Verification items for the finished model (mm, model axes). A direction names the side the tool comes from. Give positions to 0.01 mm unless a question says otherwise; leave off trailing zeros. Order: outer loops, then holes, each group sorted by start corner. A loop starts at its lowest first (then second) coordinate and runs counter-clockwise, first axis right, second up. Notation, with made-up numbers: (-22, 83.25) -> (7, 83.25) arc R24 ccw to (7, 97.25) -> close; hole circle Ø1 at (-18, -17). An arc over 180 degrees is marked (long way). Return JSON: item names as keys, results as strings. Group by question number.
(1) Cross-section at B-B on z = 88.5. Enter the section's corners in (x, y).
(2) Tool access check on faces 1 (the face through (0, -4.243, 88)), 2 (the face through (4.243, 0, 88)), 3 (the face through (0, 4.243, 88)), 4 (the face through (1.72, 4.16, 46.62)). Record the directions out of +Z, -Z, +X, -X, +Y, -Y that give a thin tool (end or side, any length) a straight path to the whole face; none if there is none.
(3) Thickness scan on line 1 along X through (y, z) = (-0.25, 52.5); line 2 along Z through (x, y) = (-5.75, -7.75); line 3 along X through (y, z) = (-2.5, 13). Record the ranges inside material, lowest first.
(4) Cross-section at D-D on z = 56.5. Enter the section's corners in (x, y), then the cut area to 3 significant figures.
(5) Depth check by flat-ended pin: pin 1 Ø3.5 at (x, z) = (-0.5, 90) entering from -Y; pin 2 Ø2.5 at (y, z) = (0.5, 88) entering from -X; pin 3 Ø8 at (y, z) = (-4.5, 62) entering from -X. Enter the tip coordinate at first touch or a pass-through.
(6) Cross-section at A-A on x = 0. Enter the section's corners in (y, z) (3 decimals), then the cut area to 3 significant figures.
from build123d import *

# Parameters (mm, degrees)
CUT_EXTRUDE_START        = -10
CUT_EXTRUDE_1_DEPTH      = 10
PATTERN_CIRCULAR_1_COUNT = 4
SCALE_1_SCALE            = 0.75


with BuildPart() as part:
    # 草图2 → 旋转1 (revolve)
    with BuildSketch(Plane(origin=(0, 0, 0), x_dir=(0, 0, -1), z_dir=(1, 0, 0))):
        Polygon((0, 0), (-143.5, 0), (-143.5, 5), (-123, 5), (-123, 6), (-3, 6), (-3, 16), (0, 16), align=None)
    revolve(axis=Axis((0, 0, 0), (0, 0, 1)))

    # 草图7 → 切除-拉伸1 (cut)
    with BuildSketch(Plane.XY.offset(123).offset(CUT_EXTRUDE_START)):
        with BuildLine():
            Line((5.656854249, 2), (5.656854249, -2))
            ThreePointArc((5.656854249, -2), (6, 0), (5.656854249, 2))
        make_face()
        with BuildLine():
            Line((-5.656854249, 2), (-5.656854249, -2))
            ThreePointArc((-5.656854249, -2), (-6, 0), (-5.656854249, 2))
        make_face()
    cut_extrude_1 = extrude(amount=CUT_EXTRUDE_1_DEPTH, mode=Mode.SUBTRACT)

    # 阵列(圆周)1: 切除-拉伸1 ×4 about axis
    pattern_circular_1_axis = Axis((0, 0, 0), (0, 0, -1))
    for i in range(1, PATTERN_CIRCULAR_1_COUNT):
        add(cut_extrude_1.rotate(pattern_circular_1_axis, i * 360 / PATTERN_CIRCULAR_1_COUNT), mode=Mode.SUBTRACT)


with BuildPart() as part_1:
    # 缩放比例1: scaled about (0, 0, 0)
    add(part.part.scale(SCALE_1_SCALE))


solid = part_1.part
Verdict:
{
 "1": {"outline": "(-4.24, -1.5) arc R4.5 ccw to (-1.5, -4.24) -> (1.5, -4.24) arc R4.5 ccw to (4.24, -1.5) -> (4.24, 1.5) arc R4.5 ccw to (1.5, 4.24) -> (-1.5, 4.24) arc R4.5 ccw to (-4.24, 1.5) -> close"},
 "2": {"face 1": "+Z, +X, -X, -Y", "face 2": "+Z, +X, +Y, -Y", "face 3": "+Z, +X, -X, +Y", "face 4": "+Z"},
 "3": {"line 1": "-4.49 to 4.49", "line 2": "0 to 2.25", "line 3": "-3.74 to 3.74"},
 "4": {"outline": "circle Ø9 at (0, 0)", "area": "63.6 mm²"},
 "5": {"pin 1": "y = -4.24", "pin 2": "x = -4.24", "pin 3": "x = -4.47"},
 "6": {"outline": "(-12, 0) -> (12, 0) -> (12, 2.25) -> (4.5, 2.25) -> (4.5, 84.75) -> (4.243, 84.75) -> (4.243, 92.25) -> (3.75, 92.25) -> (3.75, 107.625) -> (-3.75, 107.625) -> (-3.75, 92.25) -> (-4.243, 92.25) -> (-4.243, 84.75) -> (-4.5, 84.75) -> (-4.5, 2.25) -> (-12, 2.25) -> close", "area": "975 mm²"}
}
